Can you work these out from the model? Positions are in its coordinate system, mm. Face numbers are marked on the shaded views. Round coordinates to 2 decimals unless told otherwise and drop trailing zeros. Order: outer loops, then holes, each group sorted by start corner. A loop starts at its lowest first (then second) coordinate and runs counter-clockwise, first axis right, second up. Notation, with made-up numbers: (29.25, -10.5) -> (72.25, -10.5) arc R35 cw to (72.25, 25.5) -> close; hole circle Ø4 at (53.25, -19.75). An arc over 180 degrees is marked (long way). One line per item, written item: value.
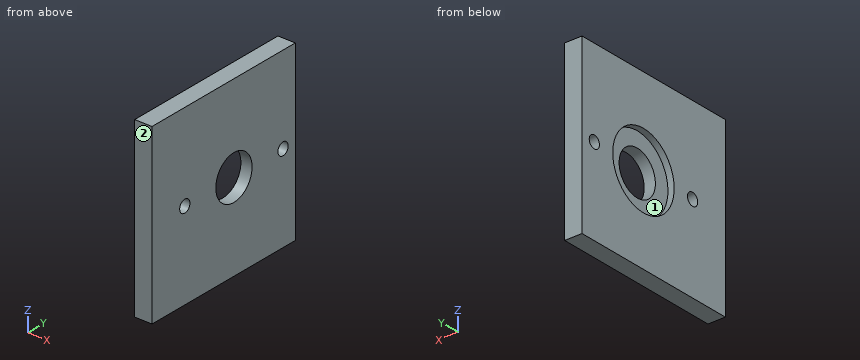
Autodesk Inventor part; units mm, degrees
ref_plane "YZ Plane" through (0, 0, 0) normal (1, 0, 0) x (0, 1, 0)
ref_plane "XZ Plane" through (0, 0, 0) normal (0, 1, 0) x (-1, 0, 0)
ref_plane "XY Plane" through (0, 0, 0) normal (0, 0, 1) x (1, 0, 0)
sketch "Sketch3" plane through (0, 0, 0) normal (1, 0, 0) x (0, 1, 0)
  line L0 (0, 0) -> (76.2, 0)
  line L1 (76.2, 0) -> (76.2, -76.2)
  line L2 (76.2, -76.2) -> (0, -76.2)
  line L3 (0, -76.2) -> (0, 0)
  line L4 (76.2, 0) -> (50.8, 0)
  line L5 (50.8, 50.8) -> (76.2, 50.8)
  line L6 (76.2, 50.8) -> (76.2, 0)
  line L7 (76.2, -76.2) -> (50.8, -76.2)
  line L8 (50.8, -127) -> (76.2, -127)
  line L9 (76.2, -127) -> (76.2, -76.2)
  line L10 (50.8, 50.8) -> (-50.8, 50.8)
  line L11 (-50.8, 50.8) -> (-50.8, 0)
  line L12 (0, 0) -> (50.8, 0)
  line L13 (50.8, -76.2) -> (0, -76.2)
  line L14 (-50.8, -76.2) -> (-50.8, -127)
  line L15 (-50.8, -127) -> (50.8, -127)
  line L16 (0, 0) -> (0, -76.2)
  line L17 (-50.8, -76.2) -> (-50.8, 0)
  dimension "d1" = 76.2
  dimension "d26" = 50.8
extrude "Extrusion1" add sketch "Sketch3" along normal blind 25.4
sketch "Sketch5" plane through (0, 0, 0) normal (-1, 0, 0) x (0, 0, 1)
  line L0 (-76.2, 76.2) -> (0, 76.2)
  line L1 (-76.2, 76.2) -> (-38.1, 76.2)
  line L2 (-38.1, 76.2) -> (-38.1, 63.5)
  line L3 (-38.1, 63.5) -> (-38.1, 38.1)
  circle A0 centre (-38.1, 38.1) radius 11.2522
  point P0 (0, 0)
  dimension "d10" = 38.1
  dimension "d11" = 12.7
  dimension "d12" = 25.4
  dimension "d13" = 22.5044
extrude "Extrusion3" cut sketch "Sketch5" against normal blind 76.2
sketch "Sketch6" plane through (25.4, 0, 0) normal (1, 0, 0) x (0, 0, -1)
  circle A0 centre (38.1, 38.1) radius 11.2522
  circle A1 centre (38.1, 38.1) radius 19.05
  point P0 (0, 0)
  dimension "d20" = 38.1
extrude "Extrusion4" cut sketch "Sketch6" against normal blind 6.35
sketch "Sketch8" plane through (0, 76.2, 50.8) normal (0, 1, 0) x (1, 0, 0)
  line L0 (0, 0) -> (25.4, 0)
  line L1 (12.7, 0) -> (9.525, 0)
  line L2 (9.525, 0) -> (15.875, 0)
  line L3 (15.875, 0) -> (15.875, 50.8)
  line L4 (15.875, 50.8) -> (9.525, 50.8)
  line L5 (9.525, 50.8) -> (9.525, 0)
  line L6 (0, 177.8) -> (0, 0)
  line L7 (12.7, 177.8) -> (9.525, 177.8)
  line L8 (9.525, 177.8) -> (15.875, 177.8)
  line L9 (15.875, 177.8) -> (15.875, 127)
  line L10 (15.875, 127) -> (9.525, 127)
  line L11 (9.525, 127) -> (9.525, 177.8)
  line L12 (0, 0) -> (0, 177.8)
  point P0 (0, 50.8)
  point P1 (25.4, 177.8)
  point P2 (15.875, 0)
  dimension "d28" = 6.35
  dimension "d29" = 50.8
extrude "Extrusion5" cut sketch "Sketch8" against normal blind 76.2
sketch "Sketch9" plane through (0, -50.8, 50.8) normal (0, 0, 1) x (1, 0, 0)
  line L0 (9.525, 50.8) -> (15.875, 50.8)
  line L1 (15.875, 50.8) -> (15.875, 0)
  line L2 (15.875, 0) -> (9.525, 0)
  line L3 (9.525, 0) -> (9.525, 50.8)
  point P0 (0, 50.8)
  dimension "d32" = 6.35
  dimension "d33" = 50.8
extrude "Extrusion6" cut sketch "Sketch9" against normal blind 203.2
sketch "Sketch10" plane through (0, 0, 0) normal (-1, 0, 0) x (0, 0, 1)
  circle A0 centre (-38.1, 38.1) radius 11.2522
  circle A1 centre (-38.1, 38.1) radius 19.05
  point P0 (0, 0)
  dimension "d36" = 38.1
extrude "Extrusion7" cut sketch "Sketch10" against normal blind 3.175 contours A0 | A1
sketch "Sketch11" plane through (0, 76.2, 50.8) normal (0, 1, 0) x (1, 0, 0)
  line L0 (9.525, 50.8) -> (15.875, 50.8)
  line L1 (16.51, 50.8) -> (16.51, 0)
  line L2 (16.51, 0) -> (8.89, 0)
  line L3 (9.525, 177.8) -> (9.525, 0)
  line L4 (8.89, 0) -> (8.89, 51.308)
  line L5 (8.89, 0) -> (60.198, 0) construction
  line L6 (8.89, 51.308) -> (16.51, 51.308)
  line L7 (16.51, 51.308) -> (16.51, 50.8)
  line L8 (0, 69.85) -> (0, 107.95)
  line L9 (0, 88.9) -> (23.8125, 88.9)
  line L10 (9.525, 127) -> (15.875, 127)
  line L11 (16.51, 127) -> (16.51, 177.8)
  line L12 (16.51, 177.8) -> (8.89, 177.8)
  line L13 (8.89, 177.8) -> (8.89, 126.492)
  line L14 (8.89, 126.492) -> (16.51, 126.492)
  line L15 (16.51, 126.492) -> (16.51, 127)
  point P0 (0, 50.8)
  point P1 (0, 127)
  dimension "d40" = 7.62
extrude "Extrusion8" cut sketch "Sketch11" against normal blind 152.4
sketch "Sketch12" plane through (25.4, -50.8, 50.8) normal (0, 0, 1) x (1, 0, 0)
  line L0 (-8.89, 127) -> (-8.89, 0)
  line L1 (-16.51, 127) -> (-16.51, 0)
  line L2 (-8.89, 50.8) -> (-16.51, 50.8)
  line L3 (-16.51, 50.8) -> (-16.51, 0)
  line L4 (-16.51, 0) -> (-8.89, 0)
  line L5 (-8.89, 0) -> (-8.89, 50.8)
  point P0 (-25.4, 50.8)
extrude "Extrusion9" cut sketch "Sketch12" against normal blind 203.2
sketch "Sketch13" plane through (25.4, 0, 0) normal (1, 0, 0) x (0, 0, -1)
  line L0 (127, 76.2) -> (-50.8, 76.2)
  line L1 (-50.8, -50.8) -> (127, -50.8)
  line L2 (-50.8, 76.2) -> (-25.4, 76.2)
  line L3 (-25.4, 76.2) -> (-25.4, -50.8)
  line L4 (-25.4, -50.8) -> (-50.8, -50.8)
  line L5 (-50.8, -50.8) -> (-50.8, 76.2)
  line L6 (127, -50.8) -> (127, 76.2)
  line L7 (127, 76.2) -> (75.692, 76.2)
  line L8 (127, -50.8) -> (101.6, -50.8)
  line L9 (101.6, -50.8) -> (101.6, 76.2)
  line L10 (101.6, 76.2) -> (127, 76.2)
  line L11 (127, 76.2) -> (127, -50.8)
  point P0 (0, 0)
  dimension "d49" = 25.4
  dimension "d50" = 25.4
extrude "Extrusion10" cut sketch "Sketch13" against normal blind 25.4 contours L6 L1 L9 L0 | L3 L1 L5 L0
sketch "Sketch14" plane through (25.4, 0, 0) normal (1, 0, 0) x (0, 0, -1)
  line L0 (-25.4, -50.8) -> (101.6, -50.8)
  line L1 (101.6, -50.8) -> (101.6, 76.2)
  line L2 (-25.4, -50.8) -> (101.6, -50.8)
  line L3 (101.6, -50.8) -> (101.6, -12.7)
  line L4 (101.6, -12.7) -> (-25.4, -12.7)
  line L5 (-25.4, -12.7) -> (-25.4, -50.8)
  point P0 (0, 0)
  dimension "d53" = 38.1
extrude "Extrusion11" cut sketch "Sketch14" against normal blind 25.4
sketch "Sketch15" plane through (25.4, 0, 0) normal (1, 0, 0) x (0, 0, -1)
  point P0 (0, 0)
sketch "Sketch16" plane through (0, 76.2, 25.4) normal (0, 0, 1) x (1, 0, 0)
  point P0 (0, -76.2)
sketch "Sketch17" plane through (8.89, 76.2, -75.692) normal (0, 1, 0) x (1, 0, 0)
  line L0 (-8.89, -101.092) -> (0, -101.092)
  line L1 (7.62, 25.908) -> (7.62, -101.092)
  line L2 (0, -101.092) -> (7.62, -101.092)
  line L3 (7.62, -101.092) -> (7.62, -62.992)
  line L4 (7.62, -62.992) -> (0, -62.992)
  line L5 (0, -62.992) -> (0, -101.092)
  line L6 (7.62, 25.908) -> (7.62, 0)
  line L7 (0, -101.092) -> (0, 25.908)
  line L8 (7.62, 25.908) -> (0, 25.908)
  line L9 (0, 25.908) -> (0, -12.192)
  line L10 (0, -12.192) -> (7.62, -12.192)
  line L11 (7.62, -12.192) -> (7.62, 25.908)
  point P0 (-8.89, -75.692)
  point P1 (7.62, -12.192)
  dimension "d56" = 38.1
  dimension "d57" = 38.1
extrude "Extrusion12" cut sketch "Sketch17" against normal blind 76.2 contours L1 L10 L7 L8 | L1 L2 L5 L4
sketch "Sketch18" plane through (8.89, 0, -12.7) normal (0, -1, 0) x (1, 0, 0)
  point P0 (-8.89, 12.7)
sketch "Sketch19" plane through (25.4, 0, 0) normal (1, 0, 0) x (0, 0, -1)
  line L0 (12.7, 76.2) -> (-25.4, 76.2)
  line L1 (-25.4, -12.7) -> (-6.35, -12.7)
  line L2 (-6.35, -12.7) -> (-6.35, 76.2)
  line L3 (-6.35, 76.2) -> (-25.4, 76.2)
  line L4 (-25.4, 76.2) -> (-25.4, -12.7)
  line L5 (101.6, -12.7) -> (-25.4, -12.7)
  line L6 (101.6, 76.2) -> (-25.4, 76.2)
  line L7 (101.6, -12.7) -> (82.55, -12.7)
  line L8 (82.55, -12.7) -> (82.55, 76.2)
  line L9 (82.55, 76.2) -> (101.6, 76.2)
  line L10 (101.6, 76.2) -> (101.6, -12.7)
  point P0 (0, 0)
  dimension "d60" = 19.05
extrude "Extrusion13" cut sketch "Sketch19" against normal blind 76.2 contours L2 L1 L4 L0 | L6 L10 L5 L8
sketch "Sketch20" plane through (0, 76.2, 6.35) normal (0, 0, 1) x (1, 0, 0)
  line L0 (8.89, -88.9) -> (0, -88.9)
  line L1 (8.89, 0) -> (8.89, -76.2)
  line L2 (0, -88.9) -> (8.89, -88.9)
  line L3 (8.89, -88.9) -> (8.89, 0)
  line L4 (8.89, 0) -> (0, 0)
  line L5 (0, 0) -> (0, -88.9)
  line L6 (16.51, 0) -> (25.4, 0)
  line L7 (8.89, -88.9) -> (8.89, 0)
  line L8 (25.4, 0) -> (8.89, 0)
  line L9 (8.89, 0) -> (8.89, -88.9)
  line L10 (8.89, -88.9) -> (25.4, -88.9)
  line L11 (25.4, -88.9) -> (25.4, 0)
  point P0 (0, -76.2)
extrude "Extrusion14" cut sketch "Sketch20" against normal blind 127 contours L3 L1 L8 L6 L11 L10
sketch "Sketch21" plane through (0, 0, 0) normal (-1, 0, 0) x (0, 0, 1)
  circle A0 centre (-38.1, 38.1) radius 11.2522
  circle A1 centre (-38.1, 68.58) radius 3.175
  circle A2 centre (-38.1, 7.62) radius 3.175
  point P0 (0, 0)
  dimension "d67" = 6.35
  dimension "d68" = 6.35
extrude "Extrusion15" cut sketch "Sketch21" against normal blind 25.4 contours A1 | A2
properties part number "220307 Rod Supports correct"
Q1. Please list where these lines run through material, in increasing order: line 1 along Y through (x, z) = (2.75, -38.1) (3 decimals); line 2 along Y through (x, z) = (7.1, -38.1) (3 decimals); line 3 along Z through (x, y) = (1.25, 8).
Answers below:
line 1: -12.7 to 4.445, 10.795 to 19.05, 57.15 to 65.405, 71.755 to 76.2
line 2: -12.7 to 4.445, 10.795 to 26.848, 49.352 to 65.405, 71.755 to 76.2
line 3: -82.55 to -41.25, -34.95 to 6.35
Q2. I want a section at B-B on y = 38.1. List the corners of the cut face in (x, z) for me (3 decimals), plus the area to 3 significant figures.
Answers below:
outline: (0, -82.55) -> (8.89, -82.55) -> (8.89, -49.352) -> (3.175, -49.352) -> (3.175, -57.15) -> (0, -57.15) -> close; (0, -19.05) -> (3.175, -19.05) -> (3.175, -26.848) -> (8.89, -26.848) -> (8.89, 6.35) -> (0, 6.35) -> close
area: 541 mm^2
Q3. I want a section at D-D on y = 68.58. List the corners of the cut face in (x, z) for me (3 decimals).
Answers below:
outline: (0, -82.55) -> (8.89, -82.55) -> (8.89, -41.275) -> (0, -41.275) -> close; (0, -34.925) -> (8.89, -34.925) -> (8.89, 6.35) -> (0, 6.35) -> close
Q4. Will these pins go through, and if not, where does the flat tip stop? pin 1 Ø7.5 at (y, z) = (7.62, -38.1) entering from -X; pin 2 Ø19 at (y, z) = (31, -38) entering from -X (3 decimals).
Answers below:
pin 1: x = 0
pin 2: x = 3.175
Q5. I want a section at A-A on x = 2. List the corners of the cut face in (y, z) for me (3 decimals).
Answers below:
outline: (-12.7, -82.55) -> (76.2, -82.55) -> (76.2, 6.35) -> (-12.7, 6.35) -> close; hole circle Ø6.35 at (7.62, -38.1); hole circle Ø38.1 at (38.1, -38.1); hole circle Ø6.35 at (68.58, -38.1)
Q6. I want a section at C-C on z = -38.1. List the corners of the cut face in (x, y) for me (3 decimals).
Answers below:
outline: (0, -12.7) -> (8.89, -12.7) -> (8.89, 4.445) -> (0, 4.445) -> close; (0, 10.795) -> (8.89, 10.795) -> (8.89, 26.848) -> (3.175, 26.848) -> (3.175, 19.05) -> (0, 19.05) -> close; (0, 57.15) -> (3.175, 57.15) -> (3.175, 49.352) -> (8.89, 49.352) -> (8.89, 65.405) -> (0, 65.405) -> close; (0, 71.755) -> (8.89, 71.755) -> (8.89, 76.2) -> (0, 76.2) -> close
Q7. We'd pull the mould along Z, two halves only. Please class the marked faces 1 and 2: released by +Z, released by -Z, zero draft, split by the parting line, or undercut.
Answers below:
face 1: undercut
face 2: zero draft
